Autodesk Inventor part; units mm, degrees
ref_plane "YZ Plane" through (0, 0, 0) normal (1, 0, 0) x (0, 1, 0)
ref_plane "XZ Plane" through (0, 0, 0) normal (0, 1, 0) x (-1, 0, 0)
ref_plane "XY Plane" through (0, 0, 0) normal (0, 0, 1) x (1, 0, 0)
sketch "Sketch1" plane through (0, 0, 0) normal (0, 1, 0) x (-1, 0, 0)
  line L0 (28, 4) -> (-28, 4)
  line L1 (-28, 4) -> (-28, -4)
  line L2 (-28, -4) -> (28, -4)
  line L3 (28, -4) -> (28, 4)
  line L4 (28, 4) -> (-28, -4) construction
  line L5 (-28, 4) -> (28, -4) construction
  point P0 (0, 0)
  dimension "d0" = 8
  dimension "d1" = 56
extrude "Extrusion1" add sketch "Sketch1" along normal blind 6
sketch "Sketch2" plane through (0, 6, 0) normal (0, 1, 0) x (1, 0, 0)
  line L0 (28, -4) -> (28, 4)
  line L1 (28, 4) -> (-28, 4)
  line L2 (-28, 4) -> (-28, -4)
  line L3 (-28, -4) -> (28, -4)
  point P0 (0, 0)
  point P1 (-17, 0)
  point P2 (-24.5, 0)
  point P3 (-9.5, 0)
  dimension "d4" = 7.5
  dimension "d5" = 11
  dimension "d14" = 7.5
hole "Hole1" at (-17, 6, 0) at (-24.5, 6, 0) at (-9.5, 6, 0) direction (0, -1, 0) diameter 4 end through all
sketch "Sketch3" plane through (0, 6, 0) normal (0, 1, 0) x (1, 0, 0)
  line L0 (28, -4) -> (28, 4)
  arc A0 (28, 0) -> (49.7378, 7.0126) centre (40, 0) ccw
  arc A1 (26, 0) -> (51.4773, 8.0169) centre (40, 0) ccw
  line L1 (51.4773, 8.0169) -> (49.7378, 7.0126)
  line L2 (28, 0) -> (28, 4)
  line L3 (28, 4) -> (-28, 4)
  line L4 (26, 4) -> (26, 0)
  point P0 (0, 0)
  dimension "d15" = 2
  dimension "d16" = 0
  dimension "d17" = 60
  dimension "d22" = 12
extrude "Extrusion2" add sketch "Sketch3" along normal blind 16 and the other way blind 6
chamfer "Chamfer1" distance 5 angle 45 2 edges at (26, 6, -2) (26.1467, 6, 2.0212)
chamfer "Chamfer2" distance 2 angle 45 2 edges at (-28, 3, 4) (-28, 3, -4)
chamfer "Chamfer3" distance 4 angle 45 3 edges at (27, 22, -4) (50.6076, 22, -7.5147) (50.6076, 0, -7.5147)
fillet "Fillet1" radius 12 1 edges at (26.5836, 3, 4)
fillet "Fillet2" radius 4 1 edges at (24.865, 8.9761, 5.2631)
properties part number "squirrely_leg_front"
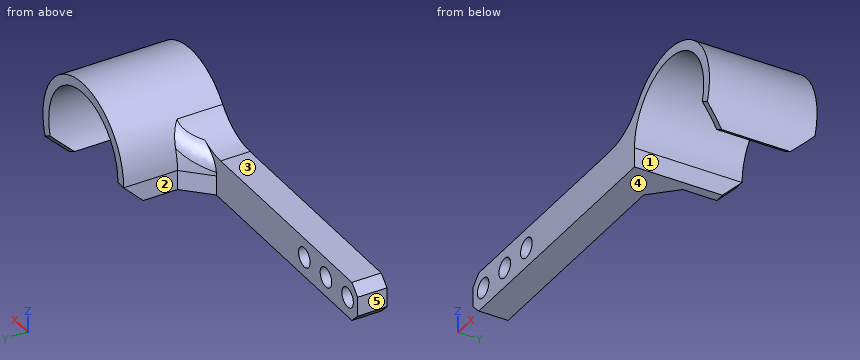
For this review, take the finished solid that the model builds, in its own axes (mm). Face numbers are marked on the shaded views. A direction names the side the tool comes from. Coordinates: 2 decimals unless noted, no trailing zeros. Loops run counter-clockwise (first coordinate to the right, second up) from the corner with the lowest first, then second, coordinate; pieces in that order, holes last. Notation, with made-up numbers: (-30.5, 1.5) - (-14.5, 1.5) arc R25 cw to (-14.5, 32.5) - close; hole circle Ø10 at (-15.5, 8.5). An arc over 180 degrees is marked (long way). Use a Markdown table: item, result. Add a question column.
Item 1: We need section C-C (x = 17). Give the boundary of the cut face in (y, z).
Item 2: We need section B-B (y = 3.25). Give the boundary of the cut face in (x, z), and give its area (3 significant figures).
Item 3: We need section A-A (x = -9.5). Give the boundary of the cut face in (y, z).
Item 4: For line 1 (X direction, y = 2.75, z = 0); line 2 (Z direction, x = -9.5, y = 1.5); line 3 (Z direction, x = 10, y = 5), list the stretches that pass through material, from the lowest coordinate up.
Item 5: Tool access review of the marked faces 4 and 5: name each direction out of +Z, -Z, +X, -X, +Y, -Y from which nothing blocks a thin tool from reaching the whole face with its end or side.
Item 6: We need section D-D (x = 44.5). Give the boundary of the cut face in (y, z).
Item 7: Insertion check: pin 1 Ø6 at (y, z) = (4.5, 6.5) entering from +X; pin 2 Ø10 at (x, z) = (8, 8.5) entering from +Y; pin 3 Ø5 at (y, z) = (14.5, 2) entering from +X; pin 4 Ø2 at (y, z) = (14, -1.5) entering from -X. Each pin has a flat end and moves straight along its axis. Give the tip position at first contact, or say it passes through.
Item 8: Mouldability with a two-part tool opening along X and no side actions: class the marked faces 1, 2 and 3 as pulls with the +X half, pulls with the -X half, needs draft (parallel to the pull), parting line crosses it, or undercut.
Results list:
| question | item | result |
|---|---|---|
| 1 | outline | (0, -4) - (6, -4) - (6, 4) - (0, 4) - close |
| 2 | outline | (-28, -2) - (-26, -4) - (28, -4) - (28, 0) arc R12 cw (long way) to (50.16, -6.39) - (51.89, -7.39) arc R14 ccw to (28.96, 8.62) arc R12 cw to (19.51, 4) - (-26, 4) - (-28, 2) - close; hole circle Ø4 at (-24.5, 0); hole circle Ø4 at (-17, 0); hole circle Ø4 at (-9.5, 0) |
| 2 | area | 502 mm^2 |
| 3 | outline | (0, -4) - (6, -4) - (6, -2) - (0, -2) - close; (0, 2) - (6, 2) - (6, 4) - (0, 4) - close |
| 4 | line 1 | x = -28 to -26.5, -22.5 to -19, -15 to -11.5, -7.5 to 28, 52 to 54 |
| 4 | line 2 | z = -4 to -2, 2 to 4 |
| 4 | line 3 | z = -4 to 4 |
| 5 | face 4 | -Z, -X, +Y, -Y |
| 5 | face 5 | +Z, -Z, -X, +Y, -Y |
| 6 | outline | (0, 11.12) - (22, 11.12) - (22, 13.26) - (0, 13.26) - close |
| 7 | pin 1 | stops at x = 53.56 |
| 7 | pin 2 | stops at y = 6 |
| 7 | pin 3 | stops at x = 54 |
| 7 | pin 4 | stops at x = 26 |
| 8 | face 1 | undercut |
| 8 | face 2 | pulls with the -X half |
| 8 | face 3 | needs draft |
